Verification items for this drawing (mm, ordinates from the low corner). A direction names the side the tool comes from. Round coordinates to 2 decimals unless told otherwise and drop trailing zeros. Order: outer loops, then holes, each group sorted by start corner. A loop starts at its lowest first (then second) coordinate and runs counter-clockwise, first axis right, second up. Notation, with made-up numbers: (74, 24.25) -> (99, 24.25) arc R17 cw to (99, 45.25) -> close; hole circle Ø10 at (89, -7.75). An arc over 180 degrees is marked (long way). Put each result on its own line as item: value.
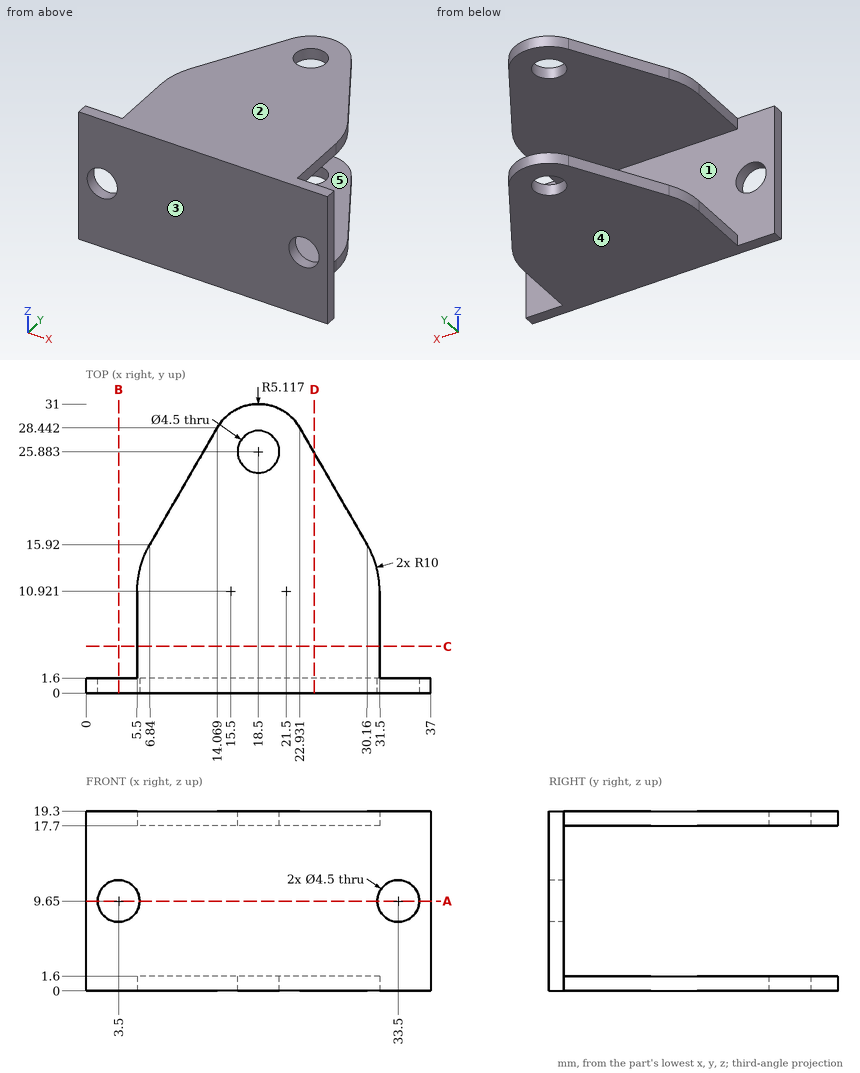
Item 1: Gauge pin test, flat ends, axial feed: pin 1 Ø6 at (x, z) = (3.5, 9.65) entering from +Y; pin 2 Ø0.8 at (y, z) = (8, 0.5) entering from -X; pin 3 Ø10 at (y, z) = (26.5, 17) entering from +X; pin 4 Ø1.5 at (y, z) = (11, 3.5) entering from +X. Record the tip position at first contact, or that the pin passes through.
Check sheet entries:
pin 1: stops at y = 1.6
pin 2: stops at x = 5.5
pin 3: stops at x = 26.91
pin 4: passes through
Item 2: Section check D-D on x = 24.5. Record the boundary of the cut face in (y, z) (1 decimal).
Check sheet entries:
outline: (0, 0) -> (25.7, 0) -> (25.7, 1.6) -> (1.6, 1.6) -> (1.6, 17.7) -> (25.7, 17.7) -> (25.7, 19.3) -> (0, 19.3) -> close
Item 3: Section check C-C on y = 5. Record the boundary of the cut face in (x, z).
Check sheet entries:
outline: (5.5, 0) -> (31.5, 0) -> (31.5, 1.6) -> (5.5, 1.6) -> close; (5.5, 17.7) -> (31.5, 17.7) -> (31.5, 19.3) -> (5.5, 19.3) -> close
Item 4: Material ranges on L1, parallel to X at y = 0.8, z = 9.65; L2, parallel to Z at x = 15, y = 15.5; L3, parallel to X at y = 1, z = 11.25, recorded low to high. Write a range as [from, to].
Check sheet entries:
L1: x = [0, 1.25], [5.75, 31.25], [35.75, 37]
L2: z = [0, 1.6], [17.7, 19.3]
L3: x = [0, 1.92], [5.08, 31.92], [35.08, 37]
Item 5: Tool access check on the marked faces 4 and 5. Record the directions out of +Z, -Z, +X, -X, +Y, -Y that give a thin tool (end or side, any length) a straight path to the whole face; none if there is none.
Check sheet entries:
face 4: -Z, +X, -X, +Y, -Y
face 5: +X, -X, +Y
Item 6: Section check B-B on x = 3.5. Record the boundary of the cut face in (y, z).
Check sheet entries:
outline: (0, 0) -> (1.6, 0) -> (1.6, 7.4) -> (0, 7.4) -> close; (0, 11.9) -> (1.6, 11.9) -> (1.6, 19.3) -> (0, 19.3) -> close
Item 7: Release check for a two-part mould opening along Z. For the marked faces 1, 2 and 3 record: +Z half, -Z half, draft (parallel to the pull), parting line (faces both ways), or undercut.
Check sheet entries:
face 1: undercut
face 2: +Z half
face 3: draft
Item 8: Section check A-A on z = 9.65. Record the boundary of the cut face in (x, y).
Check sheet entries:
outline: (0, 0) -> (1.25, 0) -> (1.25, 1.6) -> (0, 1.6) -> close; (5.75, 0) -> (31.25, 0) -> (31.25, 1.6) -> (5.75, 1.6) -> close; (35.75, 0) -> (37, 0) -> (37, 1.6) -> (35.75, 1.6) -> close
